Can you work these out from the drawing? Everything is in mm from the part's minimum corner. Round coordinates to 2 decimals unless told otherwise and drop trailing zeros. Loops run counter-clockwise (first coordinate to the right, second up) from the corner with the lowest first, then second, coordinate; pieces in that order, holes last. Notation, with made-up numbers: M 66.25,13 L 78.25,13 A11 ccw 78.25,28 Z; hole C -37.75,35 d7. An arc over 180 degrees is marked long. Use a Markdown table: item, result.
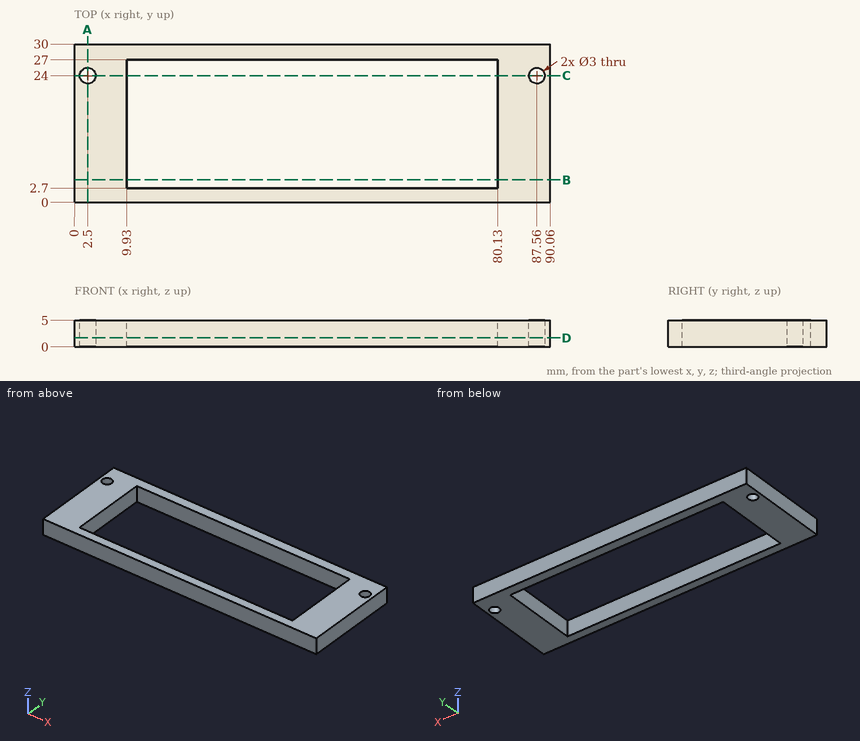
1. Imagine slicing it at D-D, the plane z = 1.7. Write out the boundary of the cut face in (x, y).
Answer sheet:
| item | result |
|---|---|
| outline | M 0,0 L 90.06,0 L 90.06,30 L 0,30 Z; hole C 2.5,24 d3; hole M 9.93,2.7 L 80.13,2.7 L 80.13,27 L 9.93,27 Z; hole C 87.56,24 d3 |
2. I need wall thicknesses on probe 1 along Y at (x, z) = (87.56, 1.55); probe 2 along X at (y, z) = (14.5, 3.85); probe 3 along Y at (x, z) = (36.5, 3.95). Which ranges of each line are inside material? Lowest first, please. Write a range as from..to.
Answer sheet:
| item | result |
|---|---|
| probe 1 | 0..22.5, 25.5..30 |
| probe 2 | 0..9.93, 80.13..90.06 |
| probe 3 | 0..2.7, 27..30 |
3. Imagine slicing it at A-A, the plane x = 2.5. Write out the boundary of the cut face in (y, z).
Answer sheet:
| item | result |
|---|---|
| outline | M 0,0 L 22.5,0 L 22.5,5 L 0,5 Z; M 25.5,0 L 30,0 L 30,5 L 25.5,5 Z |
4. Imagine slicing it at C-C, the plane y = 24. Write out the boundary of the cut face in (x, z).
Answer sheet:
| item | result |
|---|---|
| outline | M 0,0 L 1,0 L 1,5 L 0,5 Z; M 4,0 L 9.93,0 L 9.93,5 L 4,5 Z; M 80.13,0 L 86.06,0 L 86.06,5 L 80.13,5 Z; M 89.06,0 L 90.06,0 L 90.06,5 L 89.06,5 Z |
5. Imagine slicing it at B-B, the plane y = 4.25. Write out the boundary of the cut face in (x, z).
Answer sheet:
| item | result |
|---|---|
| outline | M 0,0 L 9.93,0 L 9.93,5 L 0,5 Z; M 80.13,0 L 90.06,0 L 90.06,5 L 80.13,5 Z |
